Check sheet for the modelled part. Datum: model origin and axes. Units: mm. A direction names the side the tool comes from. Round coordinates to 2 decimals unless told otherwise and drop trailing zeros. Loops run counter-clockwise (first coordinate to the right, second up) from the corner with the lowest first, then second, coordinate; pieces in that order, holes last. Notation, with made-up numbers: (54, 4) - (70, 4) arc R14 ccw to (70, 29) - close; hole circle Ø7 at (7, 80). An arc over 180 degrees is marked (long way). Return JSON: item names as keys, results as strings.
from build123d import *

# Parameters (mm, degrees)
BOSS_EXTRUDE1_DEPTH = 2000
CUT_EXTRUDE1_DEPTH  = 100
SKETCH9_R           = 50
BOSS_EXTRUDE2_DEPTH = 50
SKETCH10_W          = 0.943556428
SKETCH10_H          = 0.956350413
CUT_EXTRUDE2_DEPTH  = 1


with BuildPart() as part:
    # Sketch4 → Revolve1 (revolve)
    with BuildSketch(Plane.XY, mode=Mode.PRIVATE) as revolve1_sk:
        Polygon((150, 250), (0, 250), (0, 0), (100, 0), (100, 200), (150, 200), align=None)
    revolve(revolve1_sk.sketch.rotate(Axis((0, 250, 0), (0, -1, 0)), 180), axis=Axis((0, 250, 0), (0, -1, 0)))

    # Sketch7 → Boss-Extrude1 (add)
    with BuildSketch(Plane(origin=(0, 250, 0), x_dir=(1, 0, 0), z_dir=(0, 1, 0))):
        with BuildLine():
            Line((-75, 50), (75, 50))
            ThreePointArc((75, 50), (125, 0), (75, -50))
            Line((75, -50), (-75, -50))
            ThreePointArc((-75, -50), (-125, 0), (-75, 50))
        make_face()
    extrude(amount=BOSS_EXTRUDE1_DEPTH)

    # Sketch8 → Cut-Extrude1 (cut)
    with BuildSketch(Plane.XY.offset(50)):
        with BuildLine():
            Line((-125, 2124.5), (-125, 2250))
            Line((-125, 2250), (125, 2250))
            Line((125, 2250), (125, 2124.5))
            ThreePointArc((125, 2124.5), (0, 2249.5), (-125, 2124.5))
        make_face()
    extrude(amount=-CUT_EXTRUDE1_DEPTH, mode=Mode.SUBTRACT)

    # Sketch9 → Boss-Extrude2 (add)
    with BuildSketch(Plane.XY.offset(50)):
        with Locations(Location((0, 1963.304019878, 0), (0, 0, 180))):
            Circle(SKETCH9_R)
    extrude(amount=BOSS_EXTRUDE2_DEPTH)

    # Sketch10 → Cut-Extrude2 (cut)
    with BuildSketch(Plane.XY.offset(100)):
        with Locations((0.471778214, 1962.825844672)):
            Rectangle(SKETCH10_W, SKETCH10_H)
    extrude(amount=-CUT_EXTRUDE2_DEPTH, mode=Mode.SUBTRACT)


solid = part.part
Q1. Sectioned sample at B-B (z = -29). Enter the section's corners in (x, y), plus the area to 3 significant figures.
Answer key:
{"outline": "(-147.17, 200) - (-95.7, 200) - (-95.7, 0) - (95.7, 0) - (95.7, 200) - (147.17, 200) - (147.17, 250) - (115.73, 250) - (115.73, 2171.74) arc R125 ccw to (-115.73, 2171.74) - (-115.73, 250) - (-147.17, 250) - close", "area": "511,000 mm²"}
Q2. Depth check by flat-ended pin: P1, Ø12, axis at x = -83, y = 654, coming from the -Z side; P2, Ø10, axis at x = 96, z = -103.5, coming from the -Y side; P3, Ø1, axis at x = 56.5, z = 25, coming from the +Y side. Enter the tip coordinate at first touch or a pass-through.
Answer key:
{"P1": "stops at z = -49.96", "P2": "stops at y = 200", "P3": "stops at y = 2236.25"}
Q3. Sectioned sample at A-A (y = 2051.5). Enter the section's corners in (x, z).
Answer key:
{"outline": "(-75, -50) - (75, -50) arc R50 ccw to (75, 50) - (-75, 50) arc R50 ccw to start"}
Q4. Draft check along Y on faces 1 (the face through (98, 200, 31)), 2 (the face through (-1, 1236, -50)), 3 (the face through (1, 1236, 50)). Enter one of: released by +Y, released by -Y, zero draft, split by the parting line, or undercut.
Answer key:
{"face 1": "released by -Y", "face 2": "zero draft", "face 3": "undercut"}
Q5. Tool access check on faces 4 (the face through (124.988, 1223.428, -1.099)), 5 (the face through (-124.988, 1223.428, 1.099)), 6 (the face through (-95.38, 101.4, -30.04)), 7 (the face through (1, 1974, 100)). Record the directions out of +Z, -Z, +X, -X, +Y, -Y that give a thin tool (end or side, any length) a straight path to the whole face; none if there is none.
Answer key:
{"face 4": "+X, +Y", "face 5": "-X, +Y", "face 6": "-Y", "face 7": "+Z, +X, -X, +Y"}
Q6. Scan lines: probe 1 along Z at (x, y) = (-16.5, 614); probe 2 along Y at (x, z) = (-97.5, -98); probe 3 along Y at (x, z) = (-29, 90). Record each from-to range of solid material in increasing order. Write a range as [from, to].
Answer key:
{"probe 1": "z = [-50, 50]", "probe 2": "y = [200, 250]", "probe 3": "y = [0, 250], [1922.57, 2004.03]"}
